Design review of the part built by this model. Coordinates are the model's own, in mm. Face numbers are marked on the shaded views. A direction names the side the tool comes from. Round coordinates to 2 decimals unless told otherwise and drop trailing zeros. Loops run counter-clockwise (first coordinate to the right, second up) from the corner with the lowest first, then second, coordinate; pieces in that order, holes last. Notation, with made-up numbers: (-26.75, 82.5) - (6.25, 82.5) arc R27 cw to (6.25, 108.5) - close; hole circle Ø9 at (23.25, 46). An arc over 180 degrees is marked (long way). Return JSON: item names as keys, results as strings. Group by question number.
(1) Wall thickness on L1, parallel to Z at x = 15, y = 8.5; L2, parallel to Y at x = -8, z = 17: over which ranges is each line inside the solid? List them lowest first. Write a range as [from, to].
(2) The part is to be moulded in two halves that separate along Z. For the marked faces 6, 7 and 8, say which applies: pulls with the +Z half, pulls with the -Z half, needs draft (parallel to the pull), parting line crosses it, or undercut.
(3) We need section B-B, the plane y = 46.5. Write out the cut boundary in (x, z).
(4) We need section D-D, the plane z = 31. Write out the cut boundary in (x, y).
(5) Clearance check with flat-ended pins moving along their axes: pin 1 (16.5 mm diameter, centred on x = 7, y = 17, fed in from -Z); pin 2 (4.5 mm diameter, centred on x = 39.07, z = 22.56, fed in from +Y); pin 3 (6.5 mm diameter, centred on x = -39.07, z = -22.56, fed in from -Y); pin 4 (2 mm diameter, centred on y = -2.5, z = 11, fed in from -X). State where each tip first meets the part, or that it passes through.
(6) We need section C-C, the plane x = -30.5. Write out the cut boundary in (y, z) (3 decimals), and give its area (3 significant figures).
(7) For the marked faces 1, 2, 3, 4 and 5, list the 3-axis set-ups (+Z, -Z, +X, -X, +Y, -Y) from which the entire face can be reached by the end or side of a thin tool; tool diameter is ignored.
from build123d import *

# Parameters (mm, degrees)
SKETCH1_W                  = 55
SKETCH1_H                  = 55
SKETCH1_W_2                = 45
SKETCH1_H_2                = 45
BOSS_EXTRUDE1_DEPTH        = 5
SKETCH1_3_W                = 55
SKETCH1_3_H                = 55
SKETCH1_3_W_2              = 45
SKETCH1_3_H_2              = 45
BOSS_EXTRUDE2_DEPTH        = 60
SKETCH6_R                  = 50.8
SKETCH6_W                  = 55
SKETCH6_H                  = 55
BOSS_EXTRUDE4_DEPTH        = 10
SKETCH7_R                  = 12
BOSS_EXTRUDE5_DEPTH        = 10
F_6_0_204_DIAMETER_HOLE2_D = 5.1816
SKETCH11_R                 = 7
CUT_EXTRUDE1_DEPTH         = 10
SKETCH13_R                 = 39.439805153
SKETCH13_R_2               = 34.819805153
CUT_EXTRUDE3_DEPTH         = 2.64
FILLET2_R                  = 6.35
F_6_0_204_DIAMETER_HOLE1_D = 5.1816
CIRPATTERN2_COUNT          = 6


with BuildPart() as part:
    # Sketch1 → Boss-Extrude1 (new body)
    with BuildSketch(Plane(origin=(0, 0, 0), x_dir=(1, 0, 0), z_dir=(0, 1, 0))):
        Rectangle(SKETCH1_W, SKETCH1_H)
        Rectangle(SKETCH1_W_2, SKETCH1_H_2, mode=Mode.SUBTRACT)
        Rectangle(SKETCH1_W_2, SKETCH1_H_2)
    extrude(amount=-BOSS_EXTRUDE1_DEPTH)

    # Sketch1<3> → Boss-Extrude2 (add)
    with BuildSketch(Plane(origin=(0, 0, 0), x_dir=(1, 0, 0), z_dir=(0, 1, 0))):
        Rectangle(SKETCH1_3_W, SKETCH1_3_H)
        Rectangle(SKETCH1_3_W_2, SKETCH1_3_H_2, mode=Mode.SUBTRACT)
    extrude(amount=BOSS_EXTRUDE2_DEPTH)

    # Sketch6 → Boss-Extrude4 (add)
    with BuildSketch(Plane(origin=(0, 60, 0), x_dir=(1, 0, 0), z_dir=(0, 1, 0))):
        with Locations(Location((0, 0, 0), (0, 0, 270))):
            Circle(SKETCH6_R)
        Rectangle(SKETCH6_W, SKETCH6_H, mode=Mode.SUBTRACT)
    extrude(amount=-BOSS_EXTRUDE4_DEPTH)

    # Sketch7 → Boss-Extrude5 (add)
    with BuildSketch(Plane.XZ.offset(5)):
        with Locations(Location((0, 0, 0), (0, 0, 90))):
            Circle(SKETCH7_R)
    extrude(amount=BOSS_EXTRUDE5_DEPTH)

    # #6 (0.204) Diameter Hole2 (through all)
    with Locations(Plane(origin=(0, -15, 0), x_dir=(-1, 0, 0), z_dir=(0, -1, 0))):
        with Locations((0, 0)):
            Hole(F_6_0_204_DIAMETER_HOLE2_D / 2)

    # Sketch11 → Cut-Extrude1 (cut)
    with BuildSketch(Plane.XZ.offset(15)):
        with Locations(Location((0, 0, 0), (0, 0, 270))):
            Circle(SKETCH11_R)
    extrude(amount=-CUT_EXTRUDE1_DEPTH, mode=Mode.SUBTRACT)

    # Sketch13 → Cut-Extrude3 (cut)
    with BuildSketch(Plane(origin=(0, 60, 0), x_dir=(1, 0, 0), z_dir=(0, 1, 0))):
        with Locations(Location((0, 0, 0), (0, 0, 270))):
            Circle(SKETCH13_R)
        with Locations(Location((0, 0, 0), (0, 0, 270))):
            Circle(SKETCH13_R_2, mode=Mode.SUBTRACT)
    extrude(amount=-CUT_EXTRUDE3_DEPTH, mode=Mode.SUBTRACT)

    # Fillet2
    fillet2_edges = [part.edges().sort_by_distance(p)[0] for p in [
        (22.5, 30, 22.5),
        (-22.5, 30, 22.5),
        (-22.5, 30, -22.5),
        (22.5, 30, -22.5),
    ]]
    fillet(fillet2_edges, radius=FILLET2_R)

    # #6 (0.204) Diameter Hole1 (through all)
    with Locations(Plane(origin=(0, 60, 0), x_dir=(1, 0, 0), z_dir=(0, 1, 0))):
        with Locations((-39.074981848, -22.559951288)):
            f_6_0_204_diameter_hole1 = Hole(F_6_0_204_DIAMETER_HOLE1_D / 2)

    # CirPattern2: #6 (0.204) Diameter Hole1 ×6 about axis
    cirpattern2_axis = Axis((0, 0, 0), (0, 1, 0))
    for i in range(1, CIRPATTERN2_COUNT):
        add(f_6_0_204_diameter_hole1.rotate(cirpattern2_axis, i * 360 / CIRPATTERN2_COUNT), mode=Mode.SUBTRACT)


solid = part.part
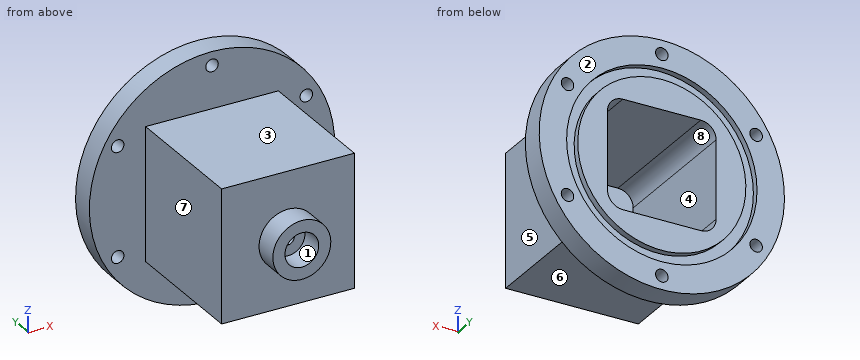
Solutions:
{
 "1": {"L1": "[-27.5, -22.5], [22.5, 27.5]", "L2": "[-5, 0]"},
 "2": {"face 6": "pulls with the -Z half", "face 7": "needs draft", "face 8": "undercut"},
 "3": {"outline": "(-27.5, -27.5) - (27.5, -27.5) - (27.5, 27.5) - (-27.5, 27.5) - close; hole (-22.5, -16.15) arc R6.35 ccw to (-16.15, -22.5) - (16.15, -22.5) arc R6.35 ccw to (22.5, -16.15) - (22.5, 16.15) arc R6.35 ccw to (16.15, 22.5) - (-16.15, 22.5) arc R6.35 ccw to (-22.5, 16.15) - close"},
 "4": {"outline": "(-40.24, 50) - (40.24, 50) - (40.24, 60) - (24.38, 60) - (24.38, 57.36) - (15.86, 57.36) - (15.86, 60) - (-15.86, 60) - (-15.86, 57.36) - (-24.38, 57.36) - (-24.38, 60) - (-40.24, 60) - close"},
 "5": {"pin 1": "z = -27.5", "pin 2": "through", "pin 3": "y = 50", "pin 4": "x = -27.5"},
 "6": {"outline": "(50, -40.625) - (60, -40.625) - (60, -25.005) - (57.36, -25.005) - (57.36, -16.798) - (60, -16.798) - (60, 16.798) - (57.36, 16.798) - (57.36, 25.005) - (60, 25.005) - (60, 40.625) - (50, 40.625) - close", "area": "769 mm^2"},
 "7": {"face 1": "-Y", "face 2": "+Z, -Z, +X, -X, +Y", "face 3": "+Z, +X, -X, -Y", "face 4": "+Y", "face 5": "+Z, -Z, +X, -Y"}
}
